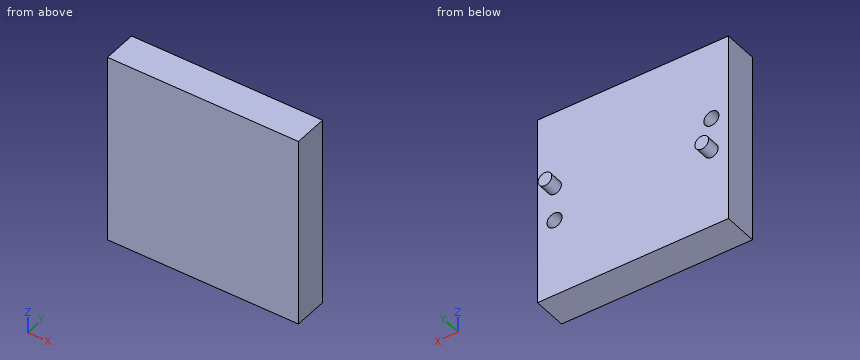
Autodesk Inventor part; units mm, degrees
ref_plane "YZ Plane" through (0, 0, 0) normal (1, 0, 0) x (0, 1, 0)
ref_plane "XZ Plane" through (0, 0, 0) normal (0, 1, 0) x (-1, 0, 0)
ref_plane "XY Plane" through (0, 0, 0) normal (0, 0, 1) x (1, 0, 0)
sketch "Sketch1" plane through (0, 0, 0) normal (0, 1, 0) x (-1, 0, 0)
  line L0 (0, -28) -> (28, -28)
  line L1 (28, 0) -> (0, 0)
  line L2 (0, 0) -> (28, 0) construction
  line L3 (0, -5) -> (0, -23)
  line L4 (28, -9) -> (28, -14)
  line L5 (23, -12) -> (23, -9)
  line L6 (23, -9) -> (28, -9)
  line L7 (28, -19) -> (28, -14)
  line L8 (23, -14) -> (23, -19)
  line L9 (23, -19) -> (28, -19)
  line L10 (28, -3) -> (28, -23)
  line L11 (28, -19) -> (28, -14)
  line L12 (28, -14) -> (28, -9)
  line L13 (28, -9) -> (28, -14)
  line L14 (28, -14) -> (28, -19)
  line L15 (28, -23) -> (28, -28)
  line L16 (28, -3) -> (28, 0)
  line L17 (14, -28) -> (14, 0)
  line L18 (0, -3) -> (0, -23)
  line L19 (0, -19) -> (0, -14)
  line L20 (5, -14) -> (5, -19)
  line L21 (5, -19) -> (0, -19)
  line L22 (0, -9) -> (0, -14)
  line L23 (5, -12) -> (5, -9)
  line L24 (5, -9) -> (0, -9)
  line L25 (0, -19) -> (0, -14)
  line L26 (0, -14) -> (0, -9)
  line L27 (0, -9) -> (0, -14)
  line L28 (0, -14) -> (0, -19)
  circle A0 centre (2.5, -16.5) radius 1.1
  circle A1 centre (2.5, -11.5) radius 1
  line L29 (0, -23) -> (0, -28)
  line L30 (0, 0) -> (0, -28)
  line L31 (25.5, -16.5) -> (28, -16.5)
  line L32 (25.5, -11.5) -> (28, -11.5)
  circle A2 centre (25.5, -16.5) radius 1
  circle A3 centre (25.5, -11.5) radius 1.1
  point P0 (25.5, -19)
  point P1 (25.5, -9)
  point P2 (23, -28)
  point P3 (23, 0)
  point P4 (23, -28)
  point P5 (23, 0)
  point P6 (2.5, -19)
  point P7 (2.5, -9)
  point P8 (28, -9)
  point P9 (0, -9)
  point P10 (28, -19)
  dimension "d18" = 5
  dimension "d20" = 2.5
  dimension "d22" = 2.5
  dimension "d25" = 2
  dimension "d26" = 2.2
  dimension "d27" = 2.2
  dimension "d28" = 28
  dimension "d29" = 28
  dimension "d36" = 28
extrude "Extrusion4" add sketch "Sketch1" along normal blind 5
extrude "Extrusion5" add sketch "Sketch1" along normal blind 7 contours A2 | A1
extrude "Extrusion6" add sketch "Sketch1" along normal blind 2.8 contours A3 | A0
properties part number "SupportoSopra"
Here's how the part is built. I have some questions about the finished solid (model axes, mm). Coordinates: 2 decimals unless noted, no trailing zeros. Order: outer loops, then holes, each group sorted by start corner. A loop starts at its lowest first (then second) coordinate and runs counter-clockwise, first axis right, second up. Notation, with made-up numbers: M -20,0.25 L -2,0.25 A10 ccw -2,17.25 Z; hole C 16.25,77 d9. An arc over 180 degrees is marked long. Answer as CSV lines item,"result".
Item 1: If I drill on line 1 (Z direction, x = -25.5, y = 4.3); line 2 (Y direction, x = -6.5, z = -26); line 3 (Z direction, x = -2.25, y = 3.75), over which ranges is the centre line in solid material (lowest first)?
Results found:
line 1,"-28 to -12.6, -10.4 to 0"
line 2,"0 to 5"
line 3,"-28 to -17.57, -15.43 to 0"
Item 2: Imagine slicing it at D-D on z = -8. Write out the boundary of the cut face in (x, y).
Results found:
outline,"M -28,0 L 0,0 L 0,5 L -28,5 Z"
Item 3: For pin 1 (0.7 mm diameter, centred on x = -25, z = -12, fed in from +Y); pin 2 (3.5 mm diameter, centred on x = -25.5, z = -11.5, fed in from +Y), each with a flat end and sliding along its axis, tell me the tip position at first contact or that it passes through.
Results found:
pin 1,"y = 2.8"
pin 2,"y = 5"
Item 4: Imagine slicing it at C-C on x = -25.5. Write out the boundary of the cut face in (y, z).
Results found:
outline,"M 0,-28 L 5,-28 L 5,-17.5 L 7,-17.5 L 7,-15.5 L 5,-15.5 L 5,-12.6 L 2.8,-12.6 L 2.8,-10.4 L 5,-10.4 L 5,0 L 0,0 Z"
Item 5: Imagine slicing it at B-B on y = 6. Write out the boundary of the cut face in (x, z), plus the area to 3 significant figures.
Results found:
outline,"C -25.5,-16.5 d2; C -2.5,-11.5 d2"
area,"6.28 mm2"
Item 6: Imagine slicing it at A-A on z = -16.5. Write out the boundary of the cut face in (x, y), plus the area to 3 significant figures.
Results found:
outline,"M -28,0 L 0,0 L 0,5 L -1.4,5 L -1.4,2.8 L -3.6,2.8 L -3.6,5 L -24.5,5 L -24.5,7 L -26.5,7 L -26.5,5 L -28,5 Z"
area,"139 mm2"
